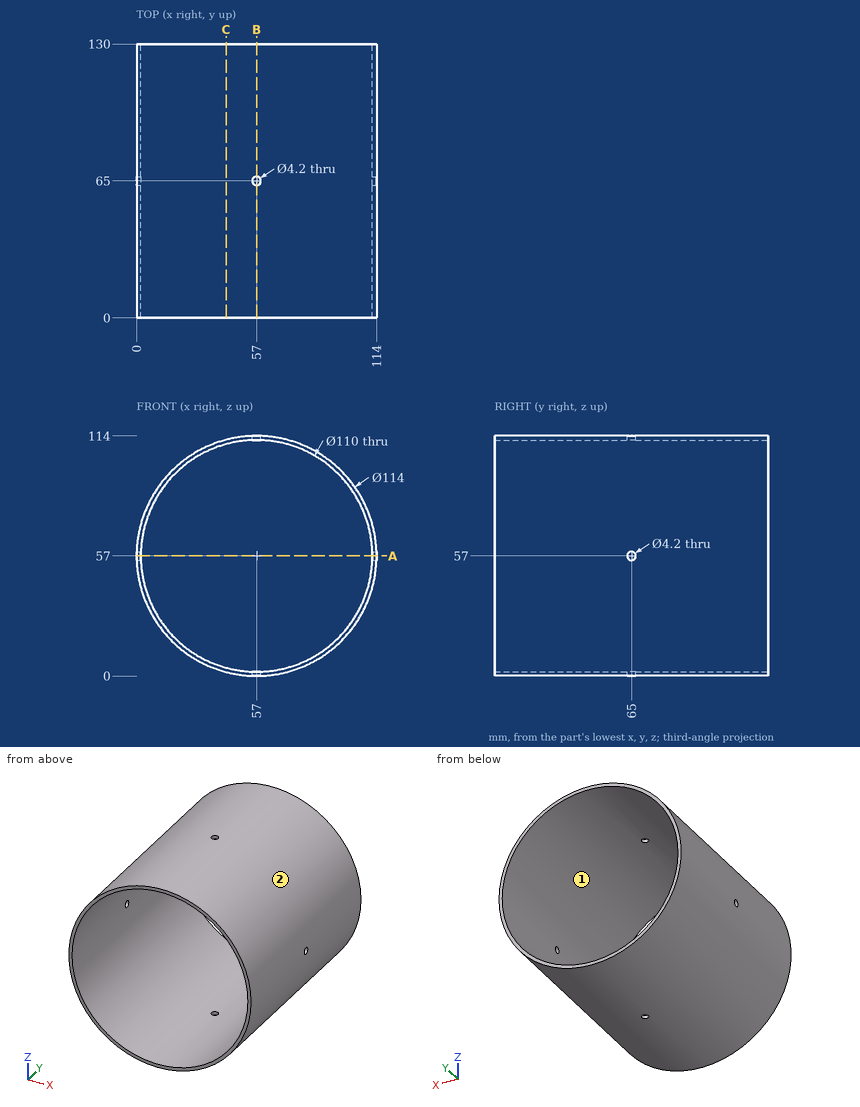
Geometry: see drawing. Coordinates: mm, zero at the bounding-box minimum. Round coordinates to 2 decimals unless told otherwise and drop trailing zeros. Loops run counter-clockwise (first coordinate to the right, second up) from the corner with the lowest first, then second, coordinate; pieces in that order, holes last. Notation, with made-up numbers: (73.25, 81) -> (128.25, 81) arc R24 cw to (128.25, 102) -> close; hole circle Ø8 at (-30.5, -7). An arc over 180 degrees is marked (long way). Write each question's results on one line, items separated by ' | '.
Item 1: Line query: probe 1 along Z at (x, y) = (57, 55); probe 2 along Y at (x, z) = (57, 1.2); probe 3 along X at (y, z) = (39.5, 30). Output: solid intervals per line, ascending. Write a range as [from, to].
Answers below:
probe 1: z = [0, 2], [112, 114] | probe 2: y = [0, 62.9], [67.1, 130] | probe 3: x = [6.8, 9.08], [104.92, 107.2]
Item 2: Cut plane A-A on z = 57. Return the cut outline in (x, y), and give its area (3 significant figures).
Answers below:
outline: (0, 0) -> (2, 0) -> (2, 62.9) -> (0, 62.9) -> close; (0, 67.1) -> (2, 67.1) -> (2, 130) -> (0, 130) -> close; (112, 0) -> (114, 0) -> (114, 62.9) -> (112, 62.9) -> close; (112, 67.1) -> (114, 67.1) -> (114, 130) -> (112, 130) -> close | area: 503 mm²
Item 3: Pull-direction query (Z, two-part tool) for the marked faces 1 and 2; classes: pulls with the +Z half, pulls with the -Z half, needs draft (parallel to the pull), parting line crosses it, or undercut.
Answers below:
face 1: undercut | face 2: parting line crosses it
Item 4: Cut plane B-B on x = 57. Return the cut outline in (y, z).
Answers below:
outline: (0, 0) -> (62.9, 0) -> (62.9, 2) -> (0, 2) -> close; (0, 112) -> (62.9, 112) -> (62.9, 114) -> (0, 114) -> close; (67.1, 0) -> (130, 0) -> (130, 2) -> (67.1, 2) -> close; (67.1, 112) -> (130, 112) -> (130, 114) -> (67.1, 114) -> close
Item 5: Cut plane C-C on x = 42.5. Return the cut outline in (y, z).
Answers below:
outline: (0, 1.88) -> (130, 1.88) -> (130, 3.95) -> (0, 3.95) -> close; (0, 110.05) -> (130, 110.05) -> (130, 112.12) -> (0, 112.12) -> close
Item 6: Pin query (flat end, axial travel): pin 1 Ø3 at (y, z) = (93, 19) entering from -X; pin 2 Ø3 at (x, y) = (61.5, 102) entering from -Z; pin 3 Ø5 at (x, y) = (22, 34) entering from -Z. Return the tip coordinate at first contact, or that it passes through.
Answers below:
pin 1: stops at x = 13.22 | pin 2: stops at z = 0.08 | pin 3: stops at z = 10.17
